```python
from build123d import *

# Parameters (mm, degrees)
BOSS_EXTRUDE1_DEPTH = 19
SKETCH4_R           = 2.55
CUT_EXTRUDE1_DEPTH  = 148.034009671
LPATTERN1_COUNT     = 6
LPATTERN1_PITCH     = 8.3
FILLET2_R           = 5
BOSS_EXTRUDE4_DEPTH = 19
BOSS_EXTRUDE5_DEPTH = 2
LPATTERN3_COUNT     = 3
LPATTERN3_PITCH     = 8.5
FILLET4_R           = 20
SKETCH9_R           = 2.15
BOSS_EXTRUDE6_DEPTH = 19
FILLET5_R           = 5


with BuildPart() as part:
    # Sketch1 → Boss-Extrude1 (new body)
    with BuildSketch(Plane(origin=(0, 0, 0), x_dir=(1, 0, 0), z_dir=(0, 1, 0))):
        with BuildLine():
            Line((0, 0), (90, 0))
            ThreePointArc((90, 0), (109.091883092, -7.908116908), (117, -27))
            Line((117, -27), (117, -87))
            Line((117, -87), (110, -87))
            Line((110, -87), (110, -27))
            ThreePointArc((110, -27), (104.142135624, -12.857864376), (90, -7))
            Line((90, -7), (0, -7))
            Line((0, -7), (0, 0))
        make_face()
    extrude(amount=BOSS_EXTRUDE1_DEPTH)

    # Sketch4 → Cut-Extrude1 (cut, through all)
    with BuildSketch(Plane(origin=(0, 0, 0), x_dir=(0, 0, -1), z_dir=(1, 0, 0))):
        with Locations((-79.5, 9)):
            Circle(SKETCH4_R)
    cut_extrude1 = extrude(amount=CUT_EXTRUDE1_DEPTH, mode=Mode.SUBTRACT)

    # LPattern1: Cut-Extrude1 ×6
    with Locations(*[(0, 0, -i * LPATTERN1_PITCH) for i in range(1, LPATTERN1_COUNT)]):
        add(cut_extrude1, mode=Mode.SUBTRACT)

    # Fillet2
    fillet2_edges = [part.edges().sort_by_distance(p)[0] for p in [
        (0, 0, 3.5),
        (113.5, 19, 87),
        (0, 19, 3.5),
        (113.5, 0, 87),
    ]]
    fillet(fillet2_edges, radius=FILLET2_R)

    # Sketch6 → Boss-Extrude4 (add)
    with BuildSketch(Plane(origin=(0, 0, 0), x_dir=(1, 0, 0), z_dir=(0, 1, 0))):
        with BuildLine():
            Line((57.067989457, 0), (96.460545107, 3))
            ThreePointArc((96.460545107, 3), (115.383129249, -6.075834674), (117, -27))
            ThreePointArc((117, -27), (109.091883092, -7.908116908), (90, 0))
            Line((90, 0), (57.067989457, 0))
        make_face()
    extrude(amount=BOSS_EXTRUDE4_DEPTH)

    # Sketch8 → Boss-Extrude5 (add)
    with BuildSketch(Plane(origin=(0, 0, 0), x_dir=(1, 0, 0), z_dir=(0, 1, 0))):
        with BuildLine():
            ThreePointArc((90, -7), (102.578584062, -14.421415938), (110, -27))
            ThreePointArc((110, -27), (104.142135624, -12.857864376), (90, -7))
        make_face()
    boss_extrude5 = extrude(amount=BOSS_EXTRUDE5_DEPTH)

    # LPattern3: Boss-Extrude5 ×3
    with Locations(*[(0, i * LPATTERN3_PITCH, 0) for i in range(1, LPATTERN3_COUNT)]):
        add(boss_extrude5)

    # Fillet4
    # the kernel refuses this fillet: 20 mm, written as the material it adds along each edge
    with BuildSketch(Plane(origin=(57.067989457, 0, 0), x_dir=(-1, 0, 0), z_dir=(0, 1, 0))) as fillet4_piece_1:
        with BuildLine():
            CenterArc((FILLET4_R * 0.0380232084134, -FILLET4_R), FILLET4_R, 90, 4.355040752)
            Line((-FILLET4_R * 0.0379134219382, -FILLET4_R * 0.00288735432207), (0, 0))
            Line((0, 0), (FILLET4_R * 0.0380232084134, 0))
        make_face()
    extrude(amount=19)

    # Sketch9 → Boss-Extrude6 (add)
    with BuildSketch(Plane.ZY.offset(-10)):
        with BuildLine():
            Line((7, 14), (12, 14))
            ThreePointArc((12, 14), (17, 9), (12, 4))
            Line((12, 4), (7, 4))
            Line((7, 4), (7, 14))
        make_face()
        with Locations((12, 9)):
            Circle(SKETCH9_R, mode=Mode.SUBTRACT)
    extrude(amount=-BOSS_EXTRUDE6_DEPTH)

    # Fillet5
    # the kernel refuses this fillet: 5 mm, written as the material it adds along each edge
    with BuildSketch(Plane(origin=(10, 4, 7), x_dir=(0, -1.0, 1.5831780331149625e-12), z_dir=(1, 0, 0))) as fillet5_piece_1:
        with BuildLine():
            CenterArc((5, -4.898979486), FILLET5_R, 101.536959033, 78.463040967)
            Line((0, -4.898979486), (0, 0))
            Line((0, 0), (4, 0))
        make_face()
    extrude(amount=19)
    with BuildSketch(Plane(origin=(10, 14, 7), x_dir=(0, 1, 0), z_dir=(1, 0, 0))) as fillet5_piece_2:
        with BuildLine():
            CenterArc((FILLET5_R, FILLET5_R), FILLET5_R, 180, 90)
            Line((0, FILLET5_R), (0, 0))
            Line((0, 0), (FILLET5_R, 0))
        make_face()
    extrude(amount=19)


solid = part.part
```
Build history of the part. All positions in model axes, mm. A direction names the side the tool comes from. Round coordinates to 2 decimals unless told otherwise and drop trailing zeros. Order: outer loops, then holes, each group sorted by start corner. A loop starts at its lowest first (then second) coordinate and runs counter-clockwise, first axis right, second up. Notation, with made-up numbers: (-33, 28.5) - (-19, 28.5) arc R4 ccw to (-19, 33.5) - close; hole circle Ø1 at (-11.5, 48.5). An arc over 180 degrees is marked (long way). Use a Markdown table: item, result.
1) Pull direction Y, two halves, no side cores. Call faces 1 (the face through (113.451, 9.112, 40.548)), 2 (the face through (96, 19, 8)), 3 (the face through (5, 9, 7)), 4 (the face through (19.367, 2.842, 8.7)): pulls with the +Y half, pulls with the -Y half, needs draft (parallel to the pull), parting line crosses it, or undercut.
Recorded:
| item | result |
|---|---|
| face 1 | undercut |
| face 2 | pulls with the +Y half |
| face 3 | needs draft |
| face 4 | pulls with the -Y half |
2) Wall check: L1, parallel to Y at x = 115, z = 38; L2, parallel to X at y = 5, z = 69; L3, parallel to X at y = 13.5, z = 11.5. Give the ranges that are in metal, low to high.
Recorded:
| item | result |
|---|---|
| L1 | y = 0 to 6.45, 11.55 to 19 |
| L2 | x = 110 to 117 |
| L3 | x = 10 to 29, 102.64 to 118.04 |
3) Saw through at C-C on z = 29. Write the cut outline in (x, y).
Recorded:
| item | result |
|---|---|
| outline | (110, 0) - (117, 0) - (117, 19) - (110, 19) - close |
4) Flat gauge pins, fed straight in: pin 1 Ø5.5 at (x, y) = (14.5, 12) entering from -Z; pin 2 Ø6.5 at (y, z) = (9, 54.6) entering from -X; pin 3 Ø4 at (y, z) = (9, 12) entering from -X. Where does each tip first touch, or does it go through?
Recorded:
| item | result |
|---|---|
| pin 1 | stops at z = 0 |
| pin 2 | stops at x = 110 |
| pin 3 | stops at x = 96.91 |
5) Saw through at A-A on z = 79.5. Write the cut outline in (x, y).
Recorded:
| item | result |
|---|---|
| outline | (110, 0) - (117, 0) - (117, 6.45) - (110, 6.45) - close; (110, 11.55) - (117, 11.55) - (117, 19) - (110, 19) - close |
6) Saw through at B-B on y = 15.25. Write the cut outline in (x, z), and give its area (3 significant figures).
Recorded:
| item | result |
|---|---|
| outline | (0.16, 0) - (56.31, 0) arc R20 cw to (57.83, -0.06) - (96.46, -3) arc R21 ccw to (117, 27) - (117, 86.84) - (110, 86.84) - (110, 27) arc R20 cw to (90, 7) - (29, 7) - (29, 8.69) - (10, 8.69) - (10, 7) - (0.16, 7) - close |
| area | 1,580 mm² |
7) Saw through at D-D on z = 45. Write the cut outline in (x, y), and give its area (3 significant figures).
Recorded:
| item | result |
|---|---|
| outline | (110, 0) - (117, 0) - (117, 6.81) - (110, 6.81) - close; (110, 11.19) - (117, 11.19) - (117, 19) - (110, 19) - close |
| area | 102 mm² |
8) Tool access for faces 5 (the face through (19.37, 10.81, 13.16)), 6 (the face through (103, 8.5, 14)), 7 (the face through (60, 9, 7)), 8 (the face through (0, 9, 4)): list every direction of +Z, -Z, +X, -X, +Y, -Y with a clear straight run to the whole face (end or side of a thin tool).
Recorded:
| item | result |
|---|---|
| face 5 | -X |
| face 6 | +Z |
| face 7 | +Z, +Y, -Y |
| face 8 | +Z, -Z, -X, +Y, -Y |
